CAD build for the part. Positions are in the model's coordinates, mm. Face numbers are marked on the shaded views. A direction names the side the tool comes from. Coordinates: 2 decimals unless noted, no trailing zeros. Loops run counter-clockwise (first coordinate to the right, second up) from the corner with the lowest first, then second, coordinate; pieces in that order, holes last.
1) Saw through at A-A, the plane z = 42. Write the cut outline in (x, y).
2) Pin check, flat tips, straight feed: pin 1 Ø10 at (x, y) = (55.5, 37.5) entering from -Z; pin 2 Ø5 at (x, y) = (40.5, 41) entering from -Z. Stop position of each tip, or through.
3) Saw through at C-C, the plane y = 27.5. Write the cut outline in (x, z), and give its area (3 significant figures).
4) Which spindle directions (+Z, -Z, +X, -X, +Y, -Y) get a long thin tool onto all of the face, cutting with end or side? Do the marked faces 5 and 6. Say none if no direction does.
5) Saw through at D-D, the plane x = 6.5. Write the cut outline in (y, z).
6) Saw through at B-B, the plane z = 25. Write the cut outline in (x, y).
7) Two-plate mould, pull along X, no slides. Class the marked faces 1, 2, 3 and 4: +X half, -X half, draft (parallel to the pull), parting line (faces both ways), or undercut.
8) Wall check: line 1 along X through (y, z) = (50, 33); line 2 along Z through (x, y) = (41, 38); line 3 along Y through (x, z) = (7, 26). Give the ranges that are in metal, low to high.
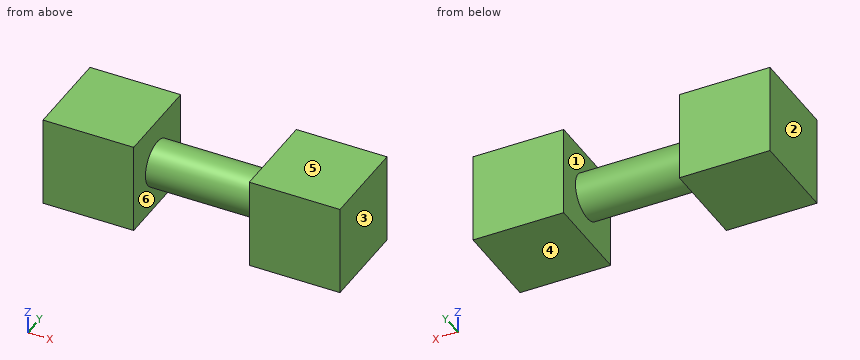
```python
from build123d import *

# Parameters (mm, degrees)
F0_W     = 50
F0_H     = 50
F1_DEPTH = 50
F2_W     = 50
F2_H     = 50
F3_DEPTH = 50
F4_R     = 12.5
F5_DEPTH = 63.726814


with BuildPart() as f1:
    # F0 (on Top) → F1 (new body)
    with BuildSketch(Plane.XY):
        with Locations((-42.158758, 37.118042)):
            Rectangle(F0_W, F0_H)
    extrude(amount=F1_DEPTH)



with BuildPart() as f3:
    # F2 (on Top) → F3 (new body, through all)
    with BuildSketch(Plane.XY):
        with Locations((71.568055, 37.118042)):
            Rectangle(F2_W, F2_H)
    extrude(amount=F3_DEPTH)


with BuildPart() as f1_1:
    add(f1.part)

    add(f3.part)  # F5 merges F3
    # F4 (on face) → F5 (join, through all)
    with BuildSketch(Plane.YZ.offset(-17.158758)):
        with Locations((37.118042, 25)):
            Circle(F4_R)
    extrude(amount=F5_DEPTH)


solid = f1_1.part
```
Data:
1. outline: (-67.16, 12.12) - (-17.16, 12.12) - (-17.16, 62.12) - (-67.16, 62.12) - close; (46.57, 12.12) - (96.57, 12.12) - (96.57, 62.12) - (46.57, 62.12) - close
2. pin 1: stops at z = 0
2. pin 2: stops at z = 12.58
3. outline: (-67.16, 0) - (-17.16, 0) - (-17.16, 17.02) - (46.57, 17.02) - (46.57, 0) - (96.57, 0) - (96.57, 50) - (46.57, 50) - (46.57, 32.98) - (-17.16, 32.98) - (-17.16, 50) - (-67.16, 50) - close
3. area: 6,020 mm2
4. face 5: +Z, +X, -X, +Y, -Y
4. face 6: none
5. outline: circle Ø25 at (37.12, 25)
6. outline: (-67.16, 12.12) - (-17.16, 12.12) - (-17.16, 24.62) - (46.57, 24.62) - (46.57, 12.12) - (96.57, 12.12) - (96.57, 62.12) - (46.57, 62.12) - (46.57, 49.62) - (-17.16, 49.62) - (-17.16, 62.12) - (-67.16, 62.12) - close
7. face 1: undercut
7. face 2: -X half
7. face 3: +X half
7. face 4: draft
8. line 1: x = -67.16 to -17.16, 46.57 to 96.57
8. line 2: z = 12.53 to 37.47
8. line 3: y = 24.66 to 49.58
